Could you check a few things on this model? Use its own coordinates, in mm. Round coordinates to 2 decimals unless told otherwise and drop trailing zeros. Write each loop counter-clockwise with the first axis right and the second up, starting at its lowest first coordinate (ties: lowest second). Pieces come first, ordered by that corner, then holes. Notation, with made-up numbers: (-14.75, 15.5) -> (-6.75, 15.5) arc R17 ccw to (-6.75, 45.5) -> close; hole circle Ø8 at (-14, -2). An arc over 180 degrees is marked (long way). Answer in a Markdown table with one row per item.
from build123d import *

# Parameters (mm, degrees)
BOSS_EXTRUDE1_DEPTH = 38.1
SKETCH2_R           = 12.7
CUT_EXTRUDE1_DEPTH  = 63.532383805
BOSS_EXTRUDE2_DEPTH = 279.4
BOSS_EXTRUDE3_DEPTH = 431.8


with BuildPart() as part:
    # Sketch1 → Boss-Extrude1 (new body)
    with BuildSketch(Plane.XY):
        Polygon((0, 0), (0, 50.8), (63.5, 0), align=None)
    extrude(amount=-BOSS_EXTRUDE1_DEPTH)

    # Sketch2 → Cut-Extrude1 (cut, through all)
    with BuildSketch(Plane(origin=(24.780487805, 30.975609756, 0), x_dir=(0.7808688094430303, -0.6246950475544244, 0), z_dir=(0.6246950475544244, 0.7808688094430304, 0))):
        with Locations(Location((7.971690031, 19.05, 0), (0, 0, 180))):
            Circle(SKETCH2_R)
    extrude(amount=-CUT_EXTRUDE1_DEPTH, mode=Mode.SUBTRACT)

    # Sketch3 → Boss-Extrude2 (add)
    with BuildSketch(Plane.XY):
        Polygon((0, 50.8), (0, 0), (63.5, 0), align=None)
    extrude(amount=BOSS_EXTRUDE2_DEPTH)

    # Sketch4 → Boss-Extrude3 (add)
    with BuildSketch(Plane(origin=(0, 0, -38.1), x_dir=(-1, 0, 0), z_dir=(0, 0, -1))):
        Polygon((0, 50.8), (-63.5, 0), (0, 0), align=None)
    extrude(amount=BOSS_EXTRUDE3_DEPTH)


solid = part.part
1) Imagine slicing it at A-A, the plane y = 42. Please give me the cut outline in (x, z), plus the area to 3 significant figures.
Findings:
| item | result |
|---|---|
| outline | (0, -469.9) -> (11, -469.9) -> (11, 279.4) -> (0, 279.4) -> close |
| area | 8,240 mm^2 |
2) Imagine slicing it at C-C, the plane z = 229. Please give me the cut outline in (x, y), plus the area to 3 significant figures.
Findings:
| item | result |
|---|---|
| outline | (0, 0) -> (63.5, 0) -> (0, 50.8) -> close |
| area | 1,610 mm^2 |
3) Imagine slicing it at B-B, the plane x = 55.5. Please give me the cut outline in (y, z).
Findings:
| item | result |
|---|---|
| outline | (0, -469.9) -> (6.4, -469.9) -> (6.4, 279.4) -> (0, 279.4) -> close |
4) For pin 1 (1 mm diameter, centred on x = 15, z = -86.5, fed in from +Y); pin 2 (3 mm diameter, centred on y = 16, z = -362, fed in from +X) (3 decimals); pin 3 (3 mm diameter, centred on y = 16.5, z = -301, fed in from +X), each with a flat end and sliding along its axis, tell me the tip position at first contact or that it passes through.
Findings:
| item | result |
|---|---|
| pin 1 | stops at y = 39.2 |
| pin 2 | stops at x = 45.375 |
| pin 3 | stops at x = 44.75 |
5) Thinking about a two-plate mould opening in Y: for faces 1 (the face through (0, 25, -90)), 2 (the face through (31, 26, -90)), 3 (the face through (12.08, 21.73, -15.24)), which applies, +Y half, -Y half, draft (parallel to the pull), parting line (faces both ways), or undercut?
Findings:
| item | result |
|---|---|
| face 1 | draft |
| face 2 | +Y half |
| face 3 | undercut |
6) Please list where these lines run through material, in increasing order: line 1 (Z direction, x = 18, y = 10); line 2 (Z direction, x = 19.5, y = 30); line 3 (X direction, y = 38, z = -100).
Findings:
| item | result |
|---|---|
| line 1 | z = -469.9 to -31.75, -6.35 to 279.4 |
| line 2 | z = -469.9 to -24.47, -13.63 to 279.4 |
| line 3 | x = 0 to 16 |
